Autodesk Fusion 360 part; units mm, degrees
sketch "Sketch1" plane through (0, 0, 0) normal (1, 0, 0) x (0, 1, 0)
  line L0 (0, 0) -> (0, 60)
  line L1 (0, 0) -> (270, 0)
  line L2 (270, 0) -> (270, 15)
  line L3 (0, 60) -> (270, 15)
  dimension "d1" = 60
  dimension "d2" = 270
  dimension "d3" = 15
extrude "Extrude1" add sketch "Sketch1" along normal blind 250
sketch "Sketch2" plane through (0, 0, 0) normal (0, 0, -1) x (1, 0, 0)
  line L0 (0, 0) -> (0, -270)
  line L1 (0, -270) -> (250, -270)
  line L2 (250, -270) -> (250, 0)
  line L3 (250, 0) -> (0, 0)
  line L4 (250, -270) -> (250, -195)
  line L5 (250, 0) -> (165, 0)
  line L6 (0, 0) -> (0, -75)
  line L7 (250, -195) -> (165, 0)
  line L8 (165, 0) -> (0, -75)
  line L9 (0, -270) -> (85, -270)
  line L10 (0, -75) -> (85, -270)
  line L11 (85, -270) -> (250, -195)
  line L12 (0, -270) -> (250, -270)
  line L13 (250, -270) -> (250, 0)
  line L14 (250, 0) -> (0, 0)
  line L15 (0, 0) -> (0, -270)
  line L16 (250, -195) -> (231.6661, -202.9917)
  line L17 (250, -195) -> (242.0083, -176.6661)
  circle A0 centre (223.6744, -184.6578) radius 4.5
  line L18 (85, -270) -> (76.7239, -251.7927)
  line L19 (85, -270) -> (103.2073, -261.7239)
  circle A1 centre (95.0579, -243.801) radius 4.5
  line L20 (0, -75) -> (82.5001, -37.4999)
  line L21 (104.0179, -84.839) -> (136.7911, -69.9421)
  circle A2 centre (71.2447, -99.7359) radius 4.5
  circle A3 centre (136.7911, -69.9421) radius 4.5
  circle A4 centre (118.0044, -202.6073) radius 4.5
  circle A5 centre (183.5508, -172.8135) radius 4.5
  circle A6 centre (95.0579, -243.801) radius 6.5
  circle A7 centre (223.6744, -184.6578) radius 6.5
  circle A8 centre (71.2447, -99.7359) radius 6.5
  circle A9 centre (136.7911, -69.9421) radius 6.5
  circle A10 centre (118.0044, -202.6073) radius 6.5
  circle A11 centre (183.5508, -172.8135) radius 6.5
  dimension "d6" = 75
  dimension "d7" = 85
  dimension "d8" = 75
  dimension "d9" = 85
  dimension "d12" = 20
  dimension "d13" = 20
  dimension "d15" = 9
  dimension "d16" = 20
  dimension "d17" = 20
  dimension "d19" = 9
  dimension "d21" = 90.623
  dimension "d22" = 52
  dimension "d23" = 36
  dimension "d24" = 36
  dimension "d25" = 9
  dimension "d26" = 9
  dimension "d27" = 113
  dimension "d28" = 113
  dimension "d29" = 9
  dimension "d30" = 9
  dimension "d33" = 13
  dimension "d34" = 13
  dimension "d35" = 13
  dimension "d36" = 13
  dimension "d37" = 13
  dimension "d38" = 13
extrude "Extrude2" cut sketch "Sketch2" against normal blind 100 contours L0 L3 L6 L8 L14 L15 L20 | L0 L1 L9 L10 L12 L15 | L2 L3 L5 L7 L13 L14 L17 | L1 L2 L4 L11 L12 L13 L19
extrude "Extrude3" cut sketch "Sketch2" against normal blind 100 contours A0 | A1 | A3 | A2 | A4 | A5
extrude "Extrude4" cut sketch "Sketch2" against normal blind 100 contours A9 | A6 | A7 | A8 | A10 | A11
extrude "Extrude5" add sketch "Sketch2" against normal blind 25 contours A7
extrude "Extrude6" cut 1 faces at (219.6356, 180.4699, 25) along direction (0, 0, -1) blind 2
extrude "Extrude7" add sketch "Sketch2" against normal blind 30 contours A11
extrude "Extrude8" cut 1 faces at (188.9248, 175.043, 30) along direction (0, 0, -1) blind 5
extrude "Extrude9" add sketch "Sketch2" against normal blind 27 contours A10
extrude "Extrude10" cut 1 faces at (117.5741, 208.413, 27) along direction (0, 0, -1) blind 5.5
extrude "Extrude11" cut 1 faces at (117.5741, 208.413, 21.5) along direction (0, 0, -1) blind 1.5
extrude "Extrude12" add sketch "Sketch2" against normal blind 15 contours A6
extrude "Extrude13" cut 1 faces at (99.5359, 247.5155, 15) along direction (0, 0, -1) blind 2
extrude "Extrude14" add sketch "Sketch2" against normal blind 40 contours A9 | A8
extrude "Extrude15" cut 1 faces at (77.0371, 100.2824, 40) along direction (0, 0, -1) blind 3
extrude "Extrude16" add 1 faces at (142.5835, 70.4886, 40) along direction (0, 0, 1) blind 2.5
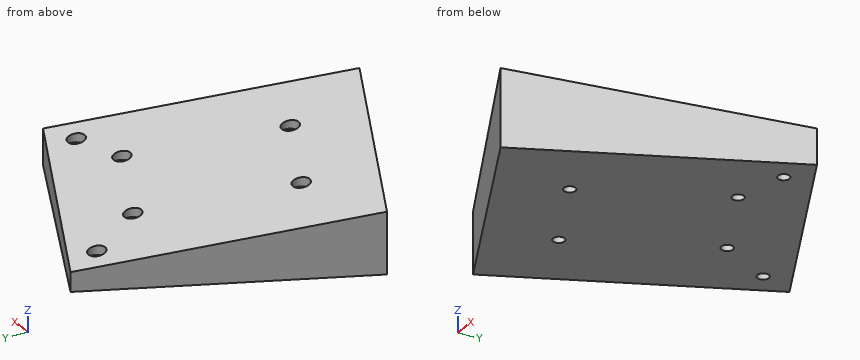
Geometry: final body of the model. Coordinates: model frame, mm. Give positions to 0.01 mm unless a question says otherwise; leave off trailing zeros. Write each loop counter-clockwise with the first axis right and the second up, starting at its lowest first coordinate (ties: lowest second). Pieces come first, ordered by that corner, then holes. Notation, with made-up numbers: (-9.5, -3.5) -> (38.5, -3.5) arc R29 cw to (38.5, 33.5) -> close; hole circle Ø1 at (71, 41). An arc over 180 degrees is marked (long way). Answer in a Markdown table with one row per item.
(1) Ray query, line 1 along X through (y, z) = (176.5, 22.5); line 2 along X through (y, z) = (174, 20.5); line 3 along Y through (x, z) = (68.5, 14.5). Return the intervals inside material, ascending. Write a range as [from, to].
Answers below:
| item | result |
|---|---|
| line 1 | [44.24, 180.97], [186.13, 241.94] |
| line 2 | [43.15, 179.21], [187.89, 240.85] |
| line 3 | [43.86, 96.17], [103.3, 232.15] |
(2) Section query A-A on y = 34.5. Return loops of the section in (x, z), then the cut area to 3 significant figures.
Answers below:
| item | result |
|---|---|
| outline | (89.1, 0) -> (180.04, 0) -> (180.04, 54.25) -> (89.1, 54.25) -> close |
| area | 4,930 mm^2 |
(3) Section query C-C on z = 52.5. Return loops of the section in (x, y).
Answers below:
| item | result |
|---|---|
| outline | (66, 45) -> (165, 0) -> (184.62, 45) -> close |
(4) Pin query (flat end, axial travel): pin 1 (17 mm diameter, centred on x = 183.55, y = 172.81, fed in from +Z) (3 decimals); pin 2 (8 mm diameter, centred on x = 118, y = 202.61, fed in from +Z); pin 3 (4 mm diameter, centred on x = 98, y = 242.5, fed in from +Z); pin 4 (4 mm diameter, centred on x = 134, y = 71, fed in from +Z). Return the tip coordinate at first contact, or that it passes through.
Answers below:
| item | result |
|---|---|
| pin 1 | z = 32.615 |
| pin 2 | through |
| pin 3 | z = 13 |
| pin 4 | z = 42.5 |
(5) Section query B-B on x = 158. Return loops of the section in (y, z).
Answers below:
| item | result |
|---|---|
| outline | (3.18, 0) -> (236.82, 0) -> (236.82, 20.53) -> (3.18, 59.47) -> close |
